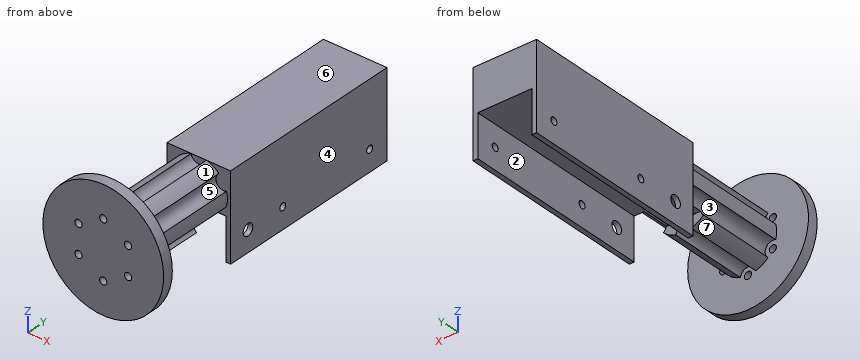
from build123d import *

# Parameters (mm, degrees)
SKETCH_1_R          = 28.5
SKETCH_1_R_2        = 1.7
EXTRUDE_1_DEPTH     = 5
SKETCH_2_R          = 13.5
EXTRUDE_2_DEPTH     = 50
SKETCH_3_R          = 3.65
CUT_EXTRUDE_1_DEPTH = 50
SKETCH_4_W          = 30
SKETCH_4_H          = 55
EXTRUDE_3_DEPTH     = 90
SKETCH_6_R          = 1.7
SKETCH_6_R_2        = 2.75
CUT_EXTRUDE_2_DEPTH = 50
SKETCH_7_W          = 25.5
SKETCH_7_H          = 110.843536678
CUT_EXTRUDE_3_DEPTH = 20
SKETCH_8_W          = 36.70966092
SKETCH_8_H          = 18.654828845
CUT_EXTRUDE_4_DEPTH = 110


with BuildPart() as part:
    # 草图1 → 凸台-拉伸1 (new body)
    with BuildSketch(Plane(origin=(0, 0, 0), x_dir=(1, 0, 0), z_dir=(0, 1, 0))):
        Circle(SKETCH_1_R)
        with Locations((0, 13.5)):
            Circle(SKETCH_1_R_2, mode=Mode.SUBTRACT)
        with Locations((11.691342951, 6.75)):
            Circle(SKETCH_1_R_2, mode=Mode.SUBTRACT)
        with Locations((11.691342951, -6.75)):
            Circle(SKETCH_1_R_2, mode=Mode.SUBTRACT)
        with Locations((0, -13.5)):
            Circle(SKETCH_1_R_2, mode=Mode.SUBTRACT)
        with Locations((-11.691342951, -6.75)):
            Circle(SKETCH_1_R_2, mode=Mode.SUBTRACT)
        with Locations((-11.691342951, 6.75)):
            Circle(SKETCH_1_R_2, mode=Mode.SUBTRACT)
    extrude(amount=EXTRUDE_1_DEPTH)

    # 草图2 → 凸台-拉伸2 (add)
    with BuildSketch(Plane(origin=(0, 5, 0), x_dir=(1, 0, 0), z_dir=(0, 1, 0))):
        Circle(SKETCH_2_R)
    extrude(amount=EXTRUDE_2_DEPTH)

    # 草图3 → 切除-拉伸1 (cut)
    with BuildSketch(Plane.XZ.offset(-5)):
        with Locations((-11.691342951, -6.75)):
            Circle(SKETCH_3_R)
        with Locations((-11.691342951, 6.75)):
            Circle(SKETCH_3_R)
        with Locations((0, 13.5)):
            Circle(SKETCH_3_R)
        with Locations((11.691342951, 6.75)):
            Circle(SKETCH_3_R)
        with Locations((11.691342951, -6.75)):
            Circle(SKETCH_3_R)
        with Locations((0, -13.5)):
            Circle(SKETCH_3_R)
    extrude(amount=-CUT_EXTRUDE_1_DEPTH, mode=Mode.SUBTRACT)

    # 草图4 → 凸台-拉伸3 (add)
    with BuildSketch(Plane(origin=(0, 55, 0), x_dir=(1, 0, 0), z_dir=(0, 1, 0))):
        Rectangle(SKETCH_4_W, SKETCH_4_H)
    extrude(amount=EXTRUDE_3_DEPTH)

    # 草图6 → 切除-拉伸2 (cut)
    with BuildSketch(Plane(origin=(15, 0, 0), x_dir=(0, 0, -1), z_dir=(1, 0, 0))):
        with Locations((17.5, 85)):
            Circle(SKETCH_6_R)
        with Locations((17.5, 135)):
            Circle(SKETCH_6_R)
        with Locations((17.5, 65)):
            Circle(SKETCH_6_R_2)
    extrude(amount=-CUT_EXTRUDE_2_DEPTH, mode=Mode.SUBTRACT)

    # 草图7 → 切除-拉伸3 (cut)
    with BuildSketch(Plane(origin=(0, 0, -27.5), x_dir=(-1, 0, 0), z_dir=(0, 0, -1))):
        with Locations((0, 97.565521138)):
            Rectangle(SKETCH_7_W, SKETCH_7_H)
    extrude(amount=-CUT_EXTRUDE_3_DEPTH, mode=Mode.SUBTRACT)

    # 草图8 → 切除-拉伸4 (cut)
    with BuildSketch(Plane.XZ.offset(-55)):
        with Locations((-1.438600971, 22.333988497)):
            Rectangle(SKETCH_8_W, SKETCH_8_H)
    extrude(amount=-CUT_EXTRUDE_4_DEPTH, mode=Mode.SUBTRACT)


solid = part.part
The listing builds one solid part. Answer for the finished solid, in the listing's coordinates (mm). Face numbers are marked on the shaded views. A direction names the side the tool comes from. Coordinates: 2 decimals unless noted, no trailing zeros. Write each loop counter-clockwise with the first axis right and the second up, starting at its lowest first coordinate (ties: lowest second). Pieces come first, ordered by that corner, then holes. Notation, with made-up numbers: (-22, 1.5) - (-5, 1.5) arc R17 cw to (-5, 20.5) - close; hole circle Ø2 at (-7.75, 68.25). An arc over 180 degrees is marked (long way). Put each result on its own line as item: value.
1. Determine the mould class of the marked faces 4, 5, 6 and 7 for opening direction Z: pulls with the +Z half, pulls with the -Z half, needs draft (parallel to the pull), parting line crosses it, or undercut.
Answer sheet:
face 4: needs draft
face 5: undercut
face 6: pulls with the +Z half
face 7: pulls with the -Z half
2. Find the intervals of material crossed by line 1 along X through (y, z) = (129.5, -8); line 2 along Z through (x, y) = (0, 3.3); line 3 along Y through (x, z) = (13, 4), in increasing order. Write a range as from..to.
Answer sheet:
line 1: x = -15..-12.75, 12.75..15
line 2: z = -28.5..-15.2, -11.8..11.8, 15.2..28.5
line 3: y = 0..5, 55..145
3. Flat-ended cylindrical pins translate along their axes: pin 1 Ø8 at (x, z) = (12, 6.5) entering from -Y; pin 2 Ø6 at (x, y) = (13.5, 119.5) entering from +Z; pin 3 Ø4.5 at (y, z) = (85, -17.5) entering from -X; pin 4 Ø12 at (y, z) = (62.5, -2.5) entering from +X. Find the tip coordinate at first contact, or state that the pin passes through.
Answer sheet:
pin 1: stops at y = 0
pin 2: stops at z = 13.01
pin 3: stops at x = -15
pin 4: stops at x = 15
4. The part is cut by section B-B on x = 0. Give the vertices of the cut face in (y, z).
Answer sheet:
outline: (0, -28.5) - (5, -28.5) - (5, -15.2) - (0, -15.2) - close; (0, -11.8) - (5, -11.8) - (5, -9.85) - (42.14, -9.85) - (42.14, -7.5) - (145, -7.5) - (145, 13.01) - (55, 13.01) - (55, 9.85) - (5, 9.85) - (5, 11.8) - (0, 11.8) - close; (0, 15.2) - (5, 15.2) - (5, 28.5) - (0, 28.5) - close
5. A tool of negligible diameter and unlimited length cuts with its end or side. For the marked faces 1, 2 and 3, from which of +Z, -Z, +X, -X, +Y, -Y can it reach the whole face along a straight path? Write none if from no direction.
Answer sheet:
face 1: +Z, +X
face 2: -Z, +Y
face 3: none
6. The part is cut by section D-D on y = 78.5. Give the vertices of the cut face in (x, z).
Answer sheet:
outline: (-15, -27.5) - (-12.75, -27.5) - (-12.75, -7.5) - (12.75, -7.5) - (12.75, -27.5) - (15, -27.5) - (15, 13.01) - (-15, 13.01) - close
7. The part is cut by section C-C on y = 27.5. Give the vertices of the cut face in (x, z), plus the area to 3 significant figures.
Answer sheet:
outline: (-13.07, -3.37) arc R3.65 cw to (-9.46, -9.64) arc R13.5 ccw to (-3.62, -13.01) arc R3.65 cw to (3.62, -13.01) arc R13.5 ccw to (9.46, -9.64) arc R3.65 cw to (13.07, -3.37) arc R13.5 ccw to (13.07, 3.37) arc R3.65 cw to (9.46, 9.64) arc R13.5 ccw to (3.62, 13.01) arc R3.65 cw to (-3.62, 13.01) arc R13.5 ccw to (-9.46, 9.64) arc R3.65 cw to (-13.07, 3.37) arc R13.5 ccw to start
area: 454 mm^2
8. The part is cut by section A-A on y = 135. Give the vertices of the cut face in (x, z), plus the area to 3 significant figures.
Answer sheet:
outline: (-15, -27.5) - (-12.75, -27.5) - (-12.75, -19.2) - (-15, -19.2) - close; (-15, -15.8) - (-12.75, -15.8) - (-12.75, -7.5) - (12.75, -7.5) - (12.75, -15.8) - (15, -15.8) - (15, 13.01) - (-15, 13.01) - close; (12.75, -27.5) - (15, -27.5) - (15, -19.2) - (12.75, -19.2) - close
area: 690 mm^2
